Could you check a few things on this model? Use its own coordinates, in mm. Give positions to 0.01 mm unless a question says otherwise; leave off trailing zeros. Write each loop counter-clockwise with the first axis right and the second up, starting at its lowest first coordinate (ties: lowest second). Pieces come first, ordered by that corner, then holes. Notation, with made-up numbers: (-1.75, 27.5) - (50.25, 27.5) arc R4 ccw to (50.25, 33.5) - close; hole circle Ø9 at (-37.75, -21). An arc over 180 degrees is marked (long way). Answer in a Markdown table with one row per item.
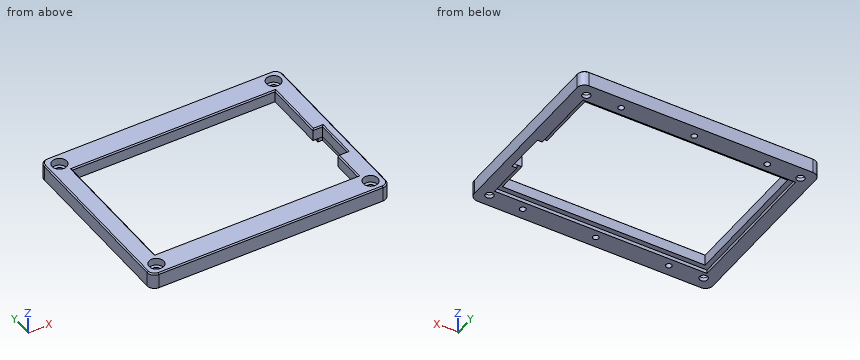
Autodesk Inventor part; units mm, degrees
ref_plane "YZ Plane" through (0, 0, 0) normal (1, 0, 0) x (0, 1, 0)
ref_plane "XZ Plane" through (0, 0, 0) normal (0, 1, 0) x (-1, 0, 0)
ref_plane "XY Plane" through (0, 0, 0) normal (0, 0, 1) x (1, 0, 0)
sketch "Sketch1" plane through (0, 0, 0) normal (0, 0, 1) x (1, 0, 0)
  line L0 (46, -37.5) -> (-46, -37.5)
  line L1 (-49, -34.5) -> (-49, 34.5)
  line L2 (-46, 37.5) -> (46, 37.5)
  line L3 (49, 34.5) -> (49, -34.5)
  line L4 (49, -37.5) -> (-49, 37.5) construction
  line L5 (-49, -37.5) -> (49, 37.5) construction
  line L6 (44, -32.5) -> (-44, -32.5) construction
  line L7 (-44, -32.5) -> (-44, 32.5) construction
  line L8 (-44, 32.5) -> (44, 32.5) construction
  line L9 (44, 32.5) -> (44, -32.5) construction
  line L10 (44, -32.5) -> (-44, 32.5) construction
  line L11 (-44, -32.5) -> (44, 32.5) construction
  arc A0 (-46, 37.5) -> (-49, 34.5) centre (-46, 34.5) ccw
  arc A1 (49, 34.5) -> (46, 37.5) centre (46, 34.5) ccw
  arc A2 (46, -37.5) -> (49, -34.5) centre (46, -34.5) ccw
  circle A3 centre (-44, 32.5) radius 1.65
  circle A4 centre (-44, -32.5) radius 1.65
  circle A5 centre (44, -32.5) radius 1.65
  circle A6 centre (44, 32.5) radius 1.65
  arc A7 (-49, -34.5) -> (-46, -37.5) centre (-46, -34.5) ccw
  point P0 (0, 0)
  dimension "d0" = 75
  dimension "d1" = 98
  dimension "d2" = 3
  dimension "d3" = 88
  dimension "d4" = 65
  dimension "d5" = 3.3
  dimension "d6" = 3
extrude "Extrusion1" add sketch "Sketch1" along normal blind 5
sketch "Sketch2" plane through (0, 0, 5) normal (0, 0, 1) x (1, 0, 0)
  line L0 (-41.65, -27.65) -> (41.65, -27.65)
  line L1 (41.65, 27.65) -> (-41.65, 27.65)
  line L2 (-41.65, 27.65) -> (-41.65, -27.65)
  line L3 (-41.65, -27.65) -> (41.65, 27.65) construction
  line L4 (41.65, -27.65) -> (-41.65, 27.65) construction
  line L5 (41.65, 2.35) -> (45.65, 2.35)
  line L6 (45.65, 2.35) -> (45.65, -14.65)
  line L7 (45.65, -14.65) -> (41.65, -14.65)
  line L8 (41.65, -27.65) -> (41.65, -14.65)
  line L9 (41.65, 2.35) -> (41.65, 27.65)
  point P0 (0, 0)
  dimension "d9" = 55.3
  dimension "d10" = 83.3
  dimension "d11" = 13
  dimension "d12" = 4
  dimension "d13" = 30
extrude "Extrusion2" cut sketch "Sketch2" against normal through all
sketch "Sketch3" plane through (0, 0, 0) normal (0, 0, -1) x (-1, 0, 0)
  line L0 (41.65, -27.65) -> (-41.65, -27.65)
  line L1 (-41.65, -27.65) -> (-41.65, -14.65)
  line L2 (-41.65, -14.65) -> (-45.65, -14.65) construction
  line L3 (-45.65, -14.65) -> (-45.65, 2.35) construction
  line L4 (-45.65, 2.35) -> (-41.65, 2.35) construction
  line L5 (-41.65, 2.35) -> (-41.65, 27.65)
  line L6 (-41.65, 27.65) -> (41.65, 27.65)
  line L7 (41.65, 27.65) -> (41.65, -27.65)
  arc A0 (-49, -34.5) -> (-46, -37.5) centre (-46, -34.5) ccw
  line L8 (46, -37.5) -> (-46, -37.5)
  arc A1 (46, -37.5) -> (49, -34.5) centre (46, -34.5) ccw
  line L9 (49, 34.5) -> (49, -34.5)
  arc A2 (49, 34.5) -> (46, 37.5) centre (46, 34.5) ccw
  line L10 (-46, 37.5) -> (46, 37.5)
  arc A3 (-46, 37.5) -> (-49, 34.5) centre (-46, 34.5) ccw
  line L11 (-49, -34.5) -> (-49, 34.5)
  circle A4 centre (-44, 32.5) radius 1.65
  circle A5 centre (-44, -32.5) radius 1.65
  circle A6 centre (44, -32.5) radius 1.65
  circle A7 centre (44, 32.5) radius 1.65
  line L12 (43.65, -29.65) -> (-43.65, -29.65)
  line L13 (-43.65, -29.65) -> (-43.65, 29.65)
  line L14 (-43.65, 29.65) -> (43.65, 29.65)
  line L15 (43.65, 29.65) -> (43.65, -29.65)
  line L16 (43.65, -29.65) -> (-43.65, 29.65) construction
  line L17 (-43.65, -29.65) -> (43.65, 29.65) construction
  point P0 (0, 0)
  dimension "d16" = 2
  dimension "d17" = 2
extrude "Extrusion3" add sketch "Sketch3" along normal blind 1.5
sketch "Sketch4" plane through (0, 0, -1.5) normal (0, 0, -1) x (-1, 0, 0)
  line L0 (30, -33) -> (-30, -33) construction
  line L1 (-30, -33) -> (-30, 33) construction
  line L2 (-30, 33) -> (30, 33) construction
  line L3 (30, 33) -> (30, -33) construction
  line L4 (30, -33) -> (-30, 33) construction
  line L5 (-30, -33) -> (30, 33) construction
  circle A0 centre (-30, 33) radius 1.2
  circle A1 centre (30, 33) radius 1.2
  circle A2 centre (-30, -33) radius 1.2
  circle A3 centre (30, -33) radius 1.2
  line L6 (46, 37.5) -> (-46, 37.5)
  circle A4 centre (0, 33) radius 1.2
  circle A5 centre (0, -33) radius 1.2
  point P0 (0, 0)
  dimension "d20" = 2.4
  dimension "d21" = 4.5
  dimension "d22" = 60
extrude "Extrusion4" cut sketch "Sketch4" against normal blind 5
sketch "Sketch5" plane through (0, 0, 0) normal (0, 0, 1) x (1, 0, 0)
  line L0 (45.65, 2.35) -> (43.65, 2.35)
  line L1 (43.65, -14.65) -> (43.65, 2.35)
  line L2 (43.65, -14.65) -> (45.65, -14.65)
  line L3 (45.65, -14.65) -> (45.65, 2.35)
  point P0 (0, 0)
extrude "Extrusion5" cut sketch "Sketch5" against normal blind 5
sketch "Sketch6" plane through (0, 0, 5) normal (0, 0, 1) x (1, 0, 0)
  circle A0 centre (-44, 32.5) radius 1.65
  circle A1 centre (-44, 32.5) radius 3
  circle A2 centre (44, 32.5) radius 1.65
  circle A3 centre (44, 32.5) radius 3
  circle A4 centre (44, -32.5) radius 1.65
  circle A5 centre (44, -32.5) radius 3
  circle A6 centre (-44, -32.5) radius 1.65
  circle A7 centre (-44, -32.5) radius 3
  point P0 (0, 0)
  dimension "d27" = 6
extrude "Extrusion6" cut sketch "Sketch6" against normal blind 3 contours A0 | A1 | A2 | A3 | A4 | A5 | A6 | A7
chamfer "Chamfer1" distance 0.5 angle 45 15 edges at (49, 0, 5) (48.1213, 36.6213, 5) (0, 37.5, 5) (-48.1213, 36.6213, 5) (-49, 0, 5) (-48.1213, -36.6213, 5) (0, -37.5, 5) (48.1213, -36.6213, 5) (45.65, -6.15, 5) (43.65, 2.35, 5) (41.65, 15, 5) (0, 27.65, 5) (0, -27.65, 5) (41.65, -21.15, 5) (-41.65, 0, 5)
properties part number "MainLid"
1) Imagine slicing it at A-A (y = 0.5). List the corners of the cut face in (x, z) for me, then the cut area to 4 significant figures.
Check values:
| item | result |
|---|---|
| outline | (-49, -1.5) - (-43.65, -1.5) - (-43.65, 0) - (-41.65, 0) - (-41.65, 4.5) - (-42.15, 5) - (-48.5, 5) - (-49, 4.5) - close; (45.65, -1.5) - (49, -1.5) - (49, 4.5) - (48.5, 5) - (46.15, 5) - (45.65, 4.5) - close |
| area | 66.05 mm2 |
2) Imagine slicing it at D-D (x = 30). List the corners of the cut face in (y, z) for me, then the cut area to 4 significant figures.
Check values:
| item | result |
|---|---|
| outline | (-37.5, -1.5) - (-34.2, -1.5) - (-34.2, 3.5) - (-31.8, 3.5) - (-31.8, -1.5) - (-29.65, -1.5) - (-29.65, 0) - (-27.65, 0) - (-27.65, 4.5) - (-28.15, 5) - (-37, 5) - (-37.5, 4.5) - close; (27.65, 0) - (29.65, 0) - (29.65, -1.5) - (31.8, -1.5) - (31.8, 3.5) - (34.2, 3.5) - (34.2, -1.5) - (37.5, -1.5) - (37.5, 4.5) - (37, 5) - (28.15, 5) - (27.65, 4.5) - close |
| area | 97.55 mm2 |
3) Imagine slicing it at C-C (y = 19). List the corners of the cut face in (x, z) for me.
Check values:
| item | result |
|---|---|
| outline | (-49, -1.5) - (-43.65, -1.5) - (-43.65, 0) - (-41.65, 0) - (-41.65, 4.5) - (-42.15, 5) - (-48.5, 5) - (-49, 4.5) - close; (41.65, 0) - (43.65, 0) - (43.65, -1.5) - (49, -1.5) - (49, 4.5) - (48.5, 5) - (42.15, 5) - (41.65, 4.5) - close |
4) Will these pins go through, and if not, where does the flat tip stop? P1, Ø1.8, axis at x = 43.5, y = -31, coming from the +Z side; P2, Ø3, axis at x = -19, y = -24.5, coming from the +Z side; P3, Ø1.4, axis at x = 0, y = 33, coming from the -Z side; P4, Ø4, axis at x = 3.5, y = 27, coming from the -Z side.
Check values:
| item | result |
|---|---|
| P1 | stops at z = 2 |
| P2 | passes through |
| P3 | stops at z = 3.5 |
| P4 | stops at z = 0 |
5) Imagine slicing it at B-B (x = 3). List the corners of the cut face in (y, z) for me.
Check values:
| item | result |
|---|---|
| outline | (-37.5, -1.5) - (-29.65, -1.5) - (-29.65, 0) - (-27.65, 0) - (-27.65, 4.5) - (-28.15, 5) - (-37, 5) - (-37.5, 4.5) - close; (27.65, 0) - (29.65, 0) - (29.65, -1.5) - (37.5, -1.5) - (37.5, 4.5) - (37, 5) - (28.15, 5) - (27.65, 4.5) - close |
6) If I drill on line 1 (Y direction, x = 0, z = 2.05); line 2 (Y direction, x = -44, z = -1); line 3 (Y direction, x = -44, z = 3), over which ranges is the centre line in solid material (lowest first)?
Check values:
| item | result |
|---|---|
| line 1 | y = -37.5 to -34.2, -31.8 to -27.65, 27.65 to 31.8, 34.2 to 37.5 |
| line 2 | y = -37.5 to -34.15, -30.85 to 30.85, 34.15 to 37.5 |
| line 3 | y = -37.5 to -35.5, -29.5 to 29.5, 35.5 to 37.5 |
